```python
from build123d import *

# Parameters (mm, degrees)
SKIZZE1_W                            = 46
SKIZZE1_H                            = 25
AUFSATZ_LINEAR_AUSTRAGEN1_DEPTH      = 3
SKIZZE3_W                            = 46
SKIZZE3_H                            = 3
AUFSATZ_LINEAR_AUSTRAGEN2_DEPTH      = 15
SCHNITT_LINEAR_AUSTRAGEN1_REACH      = 38.565
SKIZZE7_W                            = 5
SKIZZE7_H                            = 15
F_3_4_3_4_DIAMETER_HOLE2_D           = 3.4
F_3_4_3_4_DIAMETER_HOLE2_CSINK_D     = 3.45
F_3_4_3_4_DIAMETER_HOLE2_CSINK_ANGLE = 90
SCHNITT_LINEAR_AUSTRAGEN2_REACH      = 33.769
SKIZZE12_R                           = 8.05
SKIZZE12_W                           = 12
SKIZZE12_H                           = 4


with BuildPart() as part:
    # Skizze1 → Aufsatz-Linear austragen1 (new body)
    with BuildSketch(Plane(origin=(0, 0, 0), x_dir=(1, 0, 0), z_dir=(0, 1, 0))):
        Rectangle(SKIZZE1_W, SKIZZE1_H)
    extrude(amount=AUFSATZ_LINEAR_AUSTRAGEN1_DEPTH)

    # Skizze3 → Aufsatz-Linear austragen2 (add)
    with BuildSketch(Plane(origin=(0, 3, 0), x_dir=(1, 0, 0), z_dir=(0, 1, 0))):
        with Locations((0, -11)):
            Rectangle(SKIZZE3_W, SKIZZE3_H)
    extrude(amount=AUFSATZ_LINEAR_AUSTRAGEN2_DEPTH)

    # Skizze7 → Schnitt-Linear austragen1 (cut, up to next)
    with BuildSketch(Plane(origin=(0, 0, 9.5), x_dir=(-1, 0, 0), z_dir=(0, 0, -1)), mode=Mode.PRIVATE) as schnitt_linear_austragen1_sk1:
        with Locations((-20.5, 10.5)):
            Rectangle(SKIZZE7_W, SKIZZE7_H)
    schnitt_linear_austragen1_tool1 = extrude(schnitt_linear_austragen1_sk1.sketch, amount=-SCHNITT_LINEAR_AUSTRAGEN1_REACH, mode=Mode.PRIVATE) & part.part
    # Skizze7 → Schnitt-Linear austragen1 (cut, up to next)
    with BuildSketch(Plane(origin=(0, 0, 9.5), x_dir=(-1, 0, 0), z_dir=(0, 0, -1)), mode=Mode.PRIVATE) as schnitt_linear_austragen1_sk2:
        with Locations((20.5, 10.5)):
            Rectangle(SKIZZE7_W, SKIZZE7_H)
    schnitt_linear_austragen1_tool2 = extrude(schnitt_linear_austragen1_sk2.sketch, amount=-SCHNITT_LINEAR_AUSTRAGEN1_REACH, mode=Mode.PRIVATE) & part.part
    add(schnitt_linear_austragen1_tool1.solids().sort_by_distance((20.5, 10.5, 9.5))[0], mode=Mode.SUBTRACT)
    add(schnitt_linear_austragen1_tool2.solids().sort_by_distance((-20.5, 10.5, 9.5))[0], mode=Mode.SUBTRACT)

    # Ø3.4 (3.4) Diameter Hole2 (through all)
    with Locations(Plane(origin=(0, 0, 9.5), x_dir=(-1, 0, 0), z_dir=(0, 0, -1))):
        with Locations((-11.547540619, 10.006035736), (0, 10.006035736), (11.285096514, 10.006035736)):
            CounterSinkHole(F_3_4_3_4_DIAMETER_HOLE2_D / 2, F_3_4_3_4_DIAMETER_HOLE2_CSINK_D / 2, counter_sink_angle=F_3_4_3_4_DIAMETER_HOLE2_CSINK_ANGLE)

    # Skizze12 → Schnitt-Linear austragen2 (cut, up to next)
    with BuildSketch(Plane.XZ, mode=Mode.PRIVATE) as schnitt_linear_austragen2_sk1:
        with Locations(Location((-13.5, -0.5, 0), (0, 0, 270))):
            Circle(SKIZZE12_R)
    schnitt_linear_austragen2_tool1 = extrude(schnitt_linear_austragen2_sk1.sketch, amount=-SCHNITT_LINEAR_AUSTRAGEN2_REACH, mode=Mode.PRIVATE) & part.part
    # Skizze12 → Schnitt-Linear austragen2 (cut, up to next)
    with BuildSketch(Plane.XZ, mode=Mode.PRIVATE) as schnitt_linear_austragen2_sk2:
        with Locations(Location((13, -0.5, 0), (0, 0, 270))):
            Circle(SKIZZE12_R)
    schnitt_linear_austragen2_tool2 = extrude(schnitt_linear_austragen2_sk2.sketch, amount=-SCHNITT_LINEAR_AUSTRAGEN2_REACH, mode=Mode.PRIVATE) & part.part
    # Skizze12 → Schnitt-Linear austragen2 (cut, up to next)
    with BuildSketch(Plane.XZ, mode=Mode.PRIVATE) as schnitt_linear_austragen2_sk3:
        with Locations((-0.5, 7.3)):
            Rectangle(SKIZZE12_W, SKIZZE12_H)
    schnitt_linear_austragen2_tool3 = extrude(schnitt_linear_austragen2_sk3.sketch, amount=-SCHNITT_LINEAR_AUSTRAGEN2_REACH, mode=Mode.PRIVATE) & part.part
    add(schnitt_linear_austragen2_tool1.solids().sort_by_distance((-13.5, 0, -0.5))[0], mode=Mode.SUBTRACT)
    add(schnitt_linear_austragen2_tool2.solids().sort_by_distance((13, 0, -0.5))[0], mode=Mode.SUBTRACT)
    add(schnitt_linear_austragen2_tool3.solids().sort_by_distance((-0.5, 0, 7.3))[0], mode=Mode.SUBTRACT)


solid = part.part
```
Build history of the part. All positions in model axes, mm. A direction names the side the tool comes from. Give positions to 0.01 mm unless a question says otherwise; leave off trailing zeros. Loops run counter-clockwise (first coordinate to the right, second up) from the corner with the lowest first, then second, coordinate; pieces in that order, holes last.
Item 1: Slice it at A-A, the plane z = -0.5. List the corners of the cut face in (x, y), and give its area (3 significant figures).
Answers follow:
outline: (-23, 0) - (-21.55, 0) - (-21.55, 3) - (-23, 3) - close; (-5.45, 0) - (4.95, 0) - (4.95, 3) - (-5.45, 3) - close; (21.05, 0) - (23, 0) - (23, 3) - (21.05, 3) - close
area: 41.4 mm2
Item 2: Slice it at C-C, the plane x = 0. List the corners of the cut face in (y, z) (3 decimals).
Answers follow:
outline: (0, -12.5) - (3, -12.5) - (3, 5.3) - (0, 5.3) - close; (0, 9.3) - (3, 9.3) - (3, 9.5) - (8.281, 9.5) - (8.306, 9.525) - (8.306, 12.5) - (0, 12.5) - close; (11.706, 9.525) - (11.731, 9.5) - (18, 9.5) - (18, 12.5) - (11.706, 12.5) - close
Item 3: Which spindle directions (+Z, -Z, +X, -X, +Y, -Y) get a long thin tool onto all of the face, cutting with end or side? Do faces 1 (the face through (0, 12, 9.5)), 2 (the face through (5.5, 1, 7)), 3 (the face through (-0.22, 11.69, 11.03)), 4 (the face through (18, 10, 11)). Say none if no direction does.
Answers follow:
face 1: -Z, +X, -X, +Y
face 2: +Y, -Y
face 3: +Z, -Z
face 4: +Z, -Z, +X, +Y
Item 4: Slice it at B-B, the plane x = -18.5. List the corners of the cut face in (y, z), and give its area (3 significant figures).
Answers follow:
outline: (0, -12.5) - (3, -12.5) - (3, -6.81) - (0, -6.81) - close; (0, 5.81) - (3, 5.81) - (3, 12.5) - (0, 12.5) - close
area: 37.1 mm2
Item 5: Drill centre lines: line 1 (X direction, y = 1.55, z = -0.5); line 2 (Z direction, x = -8.5, y = 16.75); line 3 (Y direction, x = -1, z = -4.5). Where is each one in solid material? Low to high.
Answers follow:
line 1: x = -23 to -21.55, -5.45 to 4.95, 21.05 to 23
line 2: z = 9.5 to 12.5
line 3: y = 0 to 3
Item 6: Pull direction X, two halves, no side cores. Call faces 5 (the face through (-18, 10, 11)), 6 (the face through (-6.5, 1, 7)), 7 (the face through (-5.52, 1.48, 0.55)), 8 (the face through (0, 0, 0)): released by +X, released by -X, zero draft, split by the parting line, or undercut.
Answers follow:
face 5: released by -X
face 6: undercut
face 7: undercut
face 8: zero draft
Item 7: Flat gauge pins, fed straight in: pin 1 (3.5 mm diameter, centred on y = 12.5, z = 11.5, fed in from +X); pin 2 (8 mm diameter, centred on x = -7.5, y = 13.5, fed in from -Z); pin 3 (6 mm diameter, centred on y = 6.5, z = 0, fed in from +X); pin 4 (4 mm diameter, centred on x = 14.5, z = 7, fed in from +Y). Where does each tip first touch, or does it go through?
Answers follow:
pin 1: stops at x = 18
pin 2: stops at z = 9.5
pin 3: passes through
pin 4: stops at y = 3
Item 8: Slice it at D-D, the plane y = 13.75. List the corners of the cut face in (x, z).
Answers follow:
outline: (-18, 9.5) - (18, 9.5) - (18, 12.5) - (-18, 12.5) - close
